Could you check a few things on this model? Use its own coordinates, in mm. Face numbers are marked on the shaded views. A direction names the side the tool comes from. Give positions to 0.01 mm unless a question says otherwise; leave off trailing zeros. Write each loop counter-clockwise with the first axis right and the second up, starting at its lowest first coordinate (ties: lowest second). Pieces come first, ordered by that corner, then holes. Notation, with made-up numbers: (81.25, 22.5) - (125.25, 22.5) arc R14 ccw to (125.25, 28.5) - close; hole circle Ø1 at (-18.5, -9.5). An arc over 180 degrees is marked (long way). Use one line per item in the form item = value.
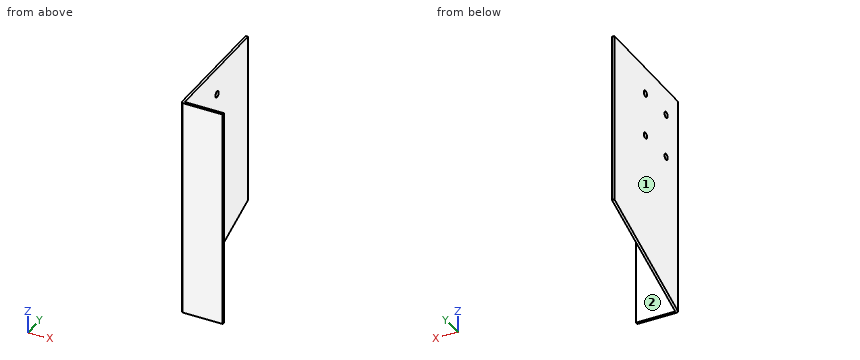
```python
from build123d import *

# Parameters (mm, degrees)
BOSS_EXTRUDE1_DEPTH = 180
FILLET1_R           = 2
SKETCH2_R           = 2.5
CUT_EXTRUDE1_DEPTH  = 180


with BuildPart() as part:
    # Sketch1 → Boss-Extrude1 (new body)
    with BuildSketch(Plane.XY):
        Polygon((-15, 50), (-15, -48), (17, -48), (17, -50), (-17, -50), (-17, 50), align=None)
    extrude(amount=BOSS_EXTRUDE1_DEPTH)

    # Fillet1
    fillet1_edges = [part.edges().sort_by_distance(p)[0] for p in [
        (-17, -50, 90),
    ]]
    fillet(fillet1_edges, radius=FILLET1_R)

    # Sketch2 → Cut-Extrude1 (cut)
    with BuildSketch(Plane.ZY.offset(17)):
        with Locations(Location((122, 2, 0), (0, 0, 270))):
            Circle(SKETCH2_R)
        with Locations(Location((122, -30, 0), (0, 0, 270))):
            Circle(SKETCH2_R)
        with Locations(Location((158, -30, 0), (0, 0, 270))):
            Circle(SKETCH2_R)
        with Locations(Location((158, 2, 0), (0, 0, 270))):
            Circle(SKETCH2_R)
        Polygon((0, -48), (39.594570132, 50), (0, 50), align=None)
    extrude(amount=-CUT_EXTRUDE1_DEPTH, mode=Mode.SUBTRACT)


solid = part.part
```
1. Imagine slicing it at A-A, the plane z = 122. List the corners of the cut face in (x, y) for me, and give its area (3 significant figures).
Response values:
outline = (-17, -48) arc R2 ccw to (-15, -50) - (17, -50) - (17, -48) - (-15, -48) - (-15, -32.5) - (-17, -32.5) - close; (-17, -27.5) - (-15, -27.5) - (-15, -0.5) - (-17, -0.5) - close; (-17, 4.5) - (-15, 4.5) - (-15, 50) - (-17, 50) - close
area = 243 mm²
2. Imagine slicing it at D-D, the plane x = 7.5. List the corners of the cut face in (y, z) for me.
Response values:
outline = (-50, 0) - (-48, 0) - (-48, 180) - (-50, 180) - close
3. For pin 1 (12 mm diameter, centred on y = -39, z = 104, fed in from +X); pin 2 (2 mm diameter, centred on x = -1.5, z = 49.5, fed in from +Y); pin 3 (4 mm diameter, centred on y = 2, z = 122, fed in from +X), each with a flat end and sliding along its axis, tell me the tip position at first contact or that it passes through.
Response values:
pin_1 = -15
pin_2 = -48
pin_3 = through
4. If I drill on line 1 (Z direction, x = -16.3, y = 2); line 2 (Z direction, x = -15.5, y = -30); line 3 (Y direction, x = -16.1, z = 158), over which ranges is the centre line in solid material (lowest first)? Write a range as from..to.
Response values:
line_1 = 20.2..119.5, 124.5..155.5, 160.5..180
line_2 = 7.27..119.5, 124.5..155.5, 160.5..180
line_3 = -49.67..-32.5, -27.5..-0.5, 4.5..50
5. Imagine slicing it at C-C, the plane z = 22.5. List the corners of the cut face in (x, y) for me.
Response values:
outline = (-17, -48) arc R2 ccw to (-15, -50) - (17, -50) - (17, -48) - (-15, -48) - (-15, 7.69) - (-17, 7.69) - close
6. Imagine slicing it at B-B, the plane y = -30. List the corners of the cut face in (x, z) for me, and give its area (3 significant figures).
Response values:
outline = (-17, 7.27) - (-15, 7.27) - (-15, 119.5) - (-17, 119.5) - close; (-17, 124.5) - (-15, 124.5) - (-15, 155.5) - (-17, 155.5) - close; (-17, 160.5) - (-15, 160.5) - (-15, 180) - (-17, 180) - close
area = 325 mm²
7. Which directions (+Z, -Z, +X, -X, +Y, -Y) give clear straight access to the entire face, cutting with the end or side of a thin tool? Please do the marked faces 1 and 2.
Response values:
face_1 = +Z, -Z, -X, +Y, -Y
face_2 = +Z, -Z, +X, +Y
